The listing builds one solid part. Answer for the finished solid, in the listing's coordinates (mm). A direction names the side the tool comes from. Round coordinates to 2 decimals unless told otherwise and drop trailing zeros. Loops run counter-clockwise (first coordinate to the right, second up) from the corner with the lowest first, then second, coordinate; pieces in that order, holes last. Notation, with made-up numbers: M 4,73 L 48,73 A13 cw 48,95 Z; hole C -31.5,-36 d7. An arc over 180 degrees is marked long. Put each result on its own line as item: value. Start each with the question number.
(1) Section B-B, the plane x = -15 is taken. Determine the outline of the cut face in (y, z), then the cut area to 3 significant figures.
(2) Section D-D, the plane y = 2.25 is taken. Count the separate pieces of the cut face and the enclosed holes in it, then the cut area to 3 significant figures.
(3) Flat-ended cylindrical pins translate along their axes: P1, Ø0.9, axis at y = 2, z = -22, coming from the -X side; P2, Ø5, axis at x = -19.5, z = -1.5, coming from the +Y side; P3, Ø1.5, axis at y = 2, z = 23, coming from the +X side; P4, Ø1.5, axis at x = -75, y = 1, coming from the +Z side. Find the tip coordinate at first contact, or state that the pin passes through.
(4) Section C-C, the plane x = -55 is taken. Determine the outline of the cut face in (y, z).
(5) Determine the mould class of faces 4 (the face through (93, 1, -102)), 5 (the face through (-1, 0, -1)), 6 (the face through (55, 1, 65)) for opening direction X: released by +X, released by -X, zero draft, split by the parting line, or undercut.
(6) Straight lines are drawn through the part: line 1 (X direction, y = 2.65, z = 29); line 2 (X direction, y = 2.25, z = -95); line 3 (X direction, y = 0.2, z = 57.5). For each, find the intervals that lie inside material, in ascending order.
(7) Section A-A, the plane z = 33 is taken. Determine the outline of the cut face in (x, y).
(8) Which of the six approach directions +Z, -Z, +X, -X, +Y, -Y give full straight-line access (tool end or side, diameter ignored) to faces 1 (the face through (-15, 1, -65)), 2 (the face through (-89.93, 1.48, 63.55)), 3 (the face through (-63.172, 1.479, -97.605))?
```python
from build123d import *

# Parameters (mm, degrees)
SKETCH_2_W          = 190
SKETCH_2_H          = 210
SKETCH_2_R          = 2
EXTRUDE_1_DEPTH     = 3
CUT_EXTRUDE_1_DEPTH = 142.629799124
CHAMFER_1_SIZE      = 5


with BuildPart() as part:
    # 草图2 → 凸台-拉伸1 (new body)
    with BuildSketch(Plane(origin=(0, 0, 0), x_dir=(1, 0, 0), z_dir=(0, 1, 0))):
        Rectangle(SKETCH_2_W, SKETCH_2_H)
        with Locations(Location((-90, 95, 0), (0, 0, 270))):
            Circle(SKETCH_2_R, mode=Mode.SUBTRACT)
        with Locations(Location((90, 95, 0), (0, 0, 90))):
            Circle(SKETCH_2_R, mode=Mode.SUBTRACT)
        with Locations(Location((90, -95, 0), (0, 0, 270))):
            Circle(SKETCH_2_R, mode=Mode.SUBTRACT)
        with Locations(Location((-90, -95, 0), (0, 0, 90))):
            Circle(SKETCH_2_R, mode=Mode.SUBTRACT)
    extrude(amount=EXTRUDE_1_DEPTH)

    # 草图3 → 切除-拉伸1 (cut, through all)
    with BuildSketch(Plane(origin=(0, 0, 0), x_dir=(1, 0, 0), z_dir=(0, 1, 0))):
        Polygon((-75.980762114, 105), (-50, 90), (50, 90), (75.980762114, 105), align=None)
        Polygon((-95, 77.474774195), (-85, 50), (-85, -50), (-95, -77.474774195), align=None)
        with BuildLine():
            Line((-50, 60), (-50, -60))
            ThreePointArc((-50, -60), (-55, -65), (-60, -60))
            Line((-60, -60), (-60, 60))
            ThreePointArc((-60, 60), (-55, 65), (-50, 60))
        make_face()
        with BuildLine():
            Line((-10, 60), (-10, -60))
            ThreePointArc((-10, -60), (-15, -65), (-20, -60))
            Line((-20, -60), (-20, 60))
            ThreePointArc((-20, 60), (-15, 65), (-10, 60))
        make_face()
        with BuildLine():
            Line((10, 60), (10, -60))
            ThreePointArc((10, -60), (15, -65), (20, -60))
            Line((20, -60), (20, 60))
            ThreePointArc((20, 60), (15, 65), (10, 60))
        make_face()
        with BuildLine():
            Line((50, 60), (50, -60))
            ThreePointArc((50, -60), (55, -65), (60, -60))
            Line((60, -60), (60, 60))
            ThreePointArc((60, 60), (55, 65), (50, 60))
        make_face()
        Polygon((85, 50), (85, -50), (95, -77.474774195), (95, 77.474774195), align=None)
        Polygon((75.980762114, -105), (50, -90), (-50, -90), (-75.980762114, -105), align=None)
    extrude(amount=CUT_EXTRUDE_1_DEPTH, mode=Mode.SUBTRACT)

    # 倒角1
    chamfer_1_edges = [part.edges().sort_by_distance(p)[0] for p in [
        (-95, 1.5, -105),
        (95, 1.5, -105),
        (95, 1.5, 105),
        (-95, 1.5, 105),
    ]]
    chamfer(chamfer_1_edges, length=CHAMFER_1_SIZE)


solid = part.part
```
Recorded:
1. outline: M 0,-90 L 3,-90 L 3,-65 L 0,-65 Z; M 0,65 L 3,65 L 3,90 L 0,90 Z
1. area: 150 mm²
2. separate pieces: 1
2. enclosed holes: 8
2. area: 28,400 mm²
3. P1: stops at x = -85
3. P2: stops at y = 3
3. P3: stops at x = 85
3. P4: stops at z = 104.87
4. outline: M 0,-92.89 L 3,-92.89 L 3,-65 L 0,-65 Z; M 0,65 L 3,65 L 3,92.89 L 0,92.89 Z
5. face 4: released by +X
5. face 5: zero draft
5. face 6: undercut
6. line 1: x = -85 to -60, -50 to -20, -10 to 10, 20 to 50, 60 to 85
6. line 2: x = -95 to -92, -88 to -58.66, 58.66 to 88, 92 to 95
6. line 3: x = -87.73 to -60, -50 to -20, -10 to 10, 20 to 50, 60 to 87.73
7. outline: M -85,0 L -60,0 L -60,3 L -85,3 Z; M -50,0 L -20,0 L -20,3 L -50,3 Z; M -10,0 L 10,0 L 10,3 L -10,3 Z; M 20,0 L 50,0 L 50,3 L 20,3 Z; M 60,0 L 85,0 L 85,3 L 60,3 Z
8. face 1: +Y, -Y
8. face 2: -X, +Y, -Y
8. face 3: -Z, +Y, -Y
